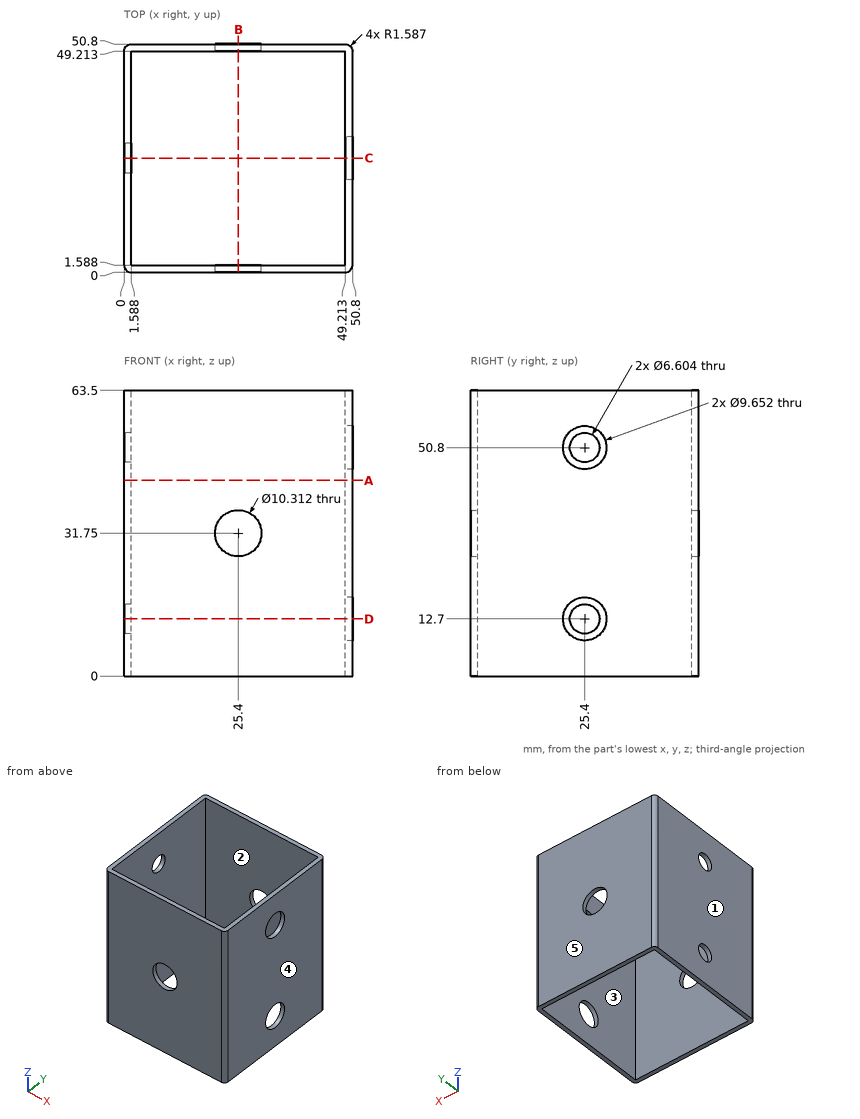
Geometry check sheet. Reference: drawing and pictorial views, mm from the part's lowest x, y, z. A direction names the side the tool comes from. Give positions to 0.01 mm unless a question says otherwise; leave off trailing zeros. Order: outer loops, then holes, each group sorted by start corner. A loop starts at its lowest first (then second) coordinate and runs counter-clockwise, first axis right, second up. Notation, with made-up numbers: (19, -11) -> (76, -11) arc R26 cw to (76, 17) -> close; hole circle Ø8 at (-6.5, -5.75). An arc over 180 degrees is marked (long way). Use CSV: the item, a comma, the result in double quotes. Start each with the question number.
1) Sectioned sample at A-A, the plane z = 43.5. Record the boundary of the cut face in (x, y) (1 decimal).
2) Set-up check for the marked faces 1 and 2: record each of +Z, -Z, +X, -X, +Y, -Y from which the full face is reachable in a straight line by a thin tool's end or side.
3) Sectioned sample at D-D, the plane z = 12.7. Record the boundary of the cut face in (x, y) (1 decimal).
4) Sectioned sample at B-B, the plane x = 25.4. Record the boundary of the cut face in (y, z).
5) Sectioned sample at C-C, the plane y = 25.4. Record the boundary of the cut face in (x, z) (1 decimal).
6) Material ranges on line 1 (Z direction, x = 0.35, y = 25.4); line 2 (Z direction, x = 49.6, y = 25.4) (1 decimal); line 3 (X direction, y = 23.5, z = 3), recorded low to high. Write a range as from..to.
7) Mould release check, pull along X, two halves, no side actions. Record for the marked faces 3, 4 and 5: released by +X, released by -X, zero draft, split by the parting line, or undercut.
Recorded:
1,outline,"(0, 1.6) arc R1.6 ccw to (1.6, 0) -> (49.2, 0) arc R1.6 ccw to (50.8, 1.6) -> (50.8, 49.2) arc R1.6 ccw to (49.2, 50.8) -> (1.6, 50.8) arc R1.6 ccw to (0, 49.2) -> close; hole (1.6, 1.6) -> (49.2, 1.6) -> (49.2, 49.2) -> (1.6, 49.2) -> close"
2,face 1,"+Z, -Z, -X, +Y, -Y"
2,face 2,"+Z, -Z"
3,outline,"(0, 1.6) arc R1.6 ccw to (1.6, 0) -> (49.2, 0) arc R1.6 ccw to (50.8, 1.6) -> (50.8, 20.6) -> (49.2, 20.6) -> (49.2, 1.6) -> (1.6, 1.6) -> (1.6, 22.1) -> (0, 22.1) -> close; (0, 28.7) -> (1.6, 28.7) -> (1.6, 49.2) -> (49.2, 49.2) -> (49.2, 30.2) -> (50.8, 30.2) -> (50.8, 49.2) arc R1.6 ccw to (49.2, 50.8) -> (1.6, 50.8) arc R1.6 ccw to (0, 49.2) -> close"
4,outline,"(0, 0) -> (1.59, 0) -> (1.59, 26.59) -> (0, 26.59) -> close; (0, 36.91) -> (1.59, 36.91) -> (1.59, 63.5) -> (0, 63.5) -> close; (49.21, 0) -> (50.8, 0) -> (50.8, 26.59) -> (49.21, 26.59) -> close; (49.21, 36.91) -> (50.8, 36.91) -> (50.8, 63.5) -> (49.21, 63.5) -> close"
5,outline,"(0, 0) -> (1.6, 0) -> (1.6, 9.4) -> (0, 9.4) -> close; (0, 16) -> (1.6, 16) -> (1.6, 47.5) -> (0, 47.5) -> close; (0, 54.1) -> (1.6, 54.1) -> (1.6, 63.5) -> (0, 63.5) -> close; (49.2, 0) -> (50.8, 0) -> (50.8, 7.9) -> (49.2, 7.9) -> close; (49.2, 17.5) -> (50.8, 17.5) -> (50.8, 46) -> (49.2, 46) -> close; (49.2, 55.6) -> (50.8, 55.6) -> (50.8, 63.5) -> (49.2, 63.5) -> close"
6,line 1,"0..9.4, 16..47.5, 54.1..63.5"
6,line 2,"0..7.9, 17.5..46, 55.6..63.5"
6,line 3,"0..1.59, 49.21..50.8"
7,face 3,"undercut"
7,face 4,"released by +X"
7,face 5,"zero draft"
